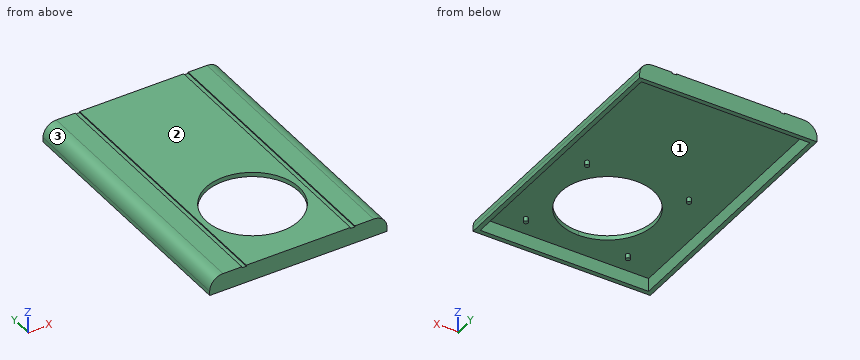
from build123d import *

# Parameters (mm, degrees)
F0_W      = 40
F0_H      = 60
F1_DEPTH  = 4
F2_W      = 1
F2_H      = 60
F3_DEPTH  = 0.25
F4_R      = 3
F6_DEPTH  = 25
F7_W      = 37.999998
F7_H      = 57.999999
F8_DEPTH  = 3
F10_DEPTH = 1


with BuildPart() as f1:
    # F0 (on Top) → F1 (new body)
    with BuildSketch(Plane.XY):
        with Locations((0, 3.187494)):
            Rectangle(F0_W, F0_H)
    extrude(amount=F1_DEPTH)

    # F2 (on face) → F3 (cut)
    with BuildSketch(Plane.XY.offset(4)):
        with Locations((-12.25, 3.187494)):
            Rectangle(F2_W, F2_H)
        with Locations((12.25, 3.187494)):
            Rectangle(F2_W, F2_H)
    extrude(amount=-F3_DEPTH, mode=Mode.SUBTRACT)

    # F4
    f4_edges = [f1.edges().sort_by_distance(p)[0] for p in [
        (-20, 3.187494, 4),
        (20, 3.187494, 4),
    ]]
    fillet(f4_edges, radius=F4_R)

    # F5 (on face) → F6 (cut)
    with BuildSketch(Plane.XY.offset(4)):
        with BuildLine():
            ThreePointArc((0, -20.812506), (7.424621, -17.737128), (10.5, -10.312506))
            ThreePointArc((10.5, -10.312506), (-7.424621, -2.887885), (0, -20.812506))
        make_face()
    extrude(amount=-F6_DEPTH, mode=Mode.SUBTRACT)

    # F7 (on face) → F8 (cut)
    with BuildSketch(Plane(origin=(0, 0, 0), x_dir=(1, 0, 0), z_dir=(0, 0, -1))):
        with Locations((0, -3.187493)):
            Rectangle(F7_W, F7_H)
    extrude(amount=-F8_DEPTH, mode=Mode.SUBTRACT)

    # F9 (on face) → F10 (join)
    with BuildSketch(Plane(origin=(0, 0, 3), x_dir=(1, 0, 0), z_dir=(0, 0, -1))):
        with BuildLine():
            Line((11.5, 21.312506), (11, 21.312506))
            ThreePointArc((11, 21.312506), (11.146447, 20.958953), (11.5, 20.812506))
            Line((11.5, 20.812506), (11.5, 21.312506))
        make_face()
        with BuildLine():
            ThreePointArc((12, 21.312506), (11.5, 21.812506), (11, 21.312506))
            Line((11, 21.312506), (11.5, 21.312506))
            Line((11.5, 21.312506), (11.5, 20.812506))
            ThreePointArc((11.5, 20.812506), (11.853553, 20.958953), (12, 21.312506))
        make_face()
        with BuildLine():
            Line((-11.5, 21.312506), (-11, 21.312506))
            ThreePointArc((-11, 21.312506), (-11.853553, 21.66606), (-11.5, 20.812506))
            Line((-11.5, 20.812506), (-11.5, 21.312506))
        make_face()
        with BuildLine():
            ThreePointArc((-11.5, 20.812506), (-11.146447, 20.958953), (-11, 21.312506))
            Line((-11, 21.312506), (-11.5, 21.312506))
            Line((-11.5, 21.312506), (-11.5, 20.812506))
        make_face()
        with BuildLine():
            Line((11.5, -0.687494), (11.5, -0.187494))
            ThreePointArc((11.5, -0.187494), (11.146447, -0.33394), (11, -0.687494))
            Line((11, -0.687494), (11.5, -0.687494))
        make_face()
        with BuildLine():
            ThreePointArc((12, -0.687494), (11.853553, -0.33394), (11.5, -0.187494))
            Line((11.5, -0.187494), (11.5, -0.687494))
            Line((11.5, -0.687494), (11, -0.687494))
            ThreePointArc((11, -0.687494), (11.5, -1.187494), (12, -0.687494))
        make_face()
        with BuildLine():
            ThreePointArc((-11, -0.687494), (-11.146447, -0.33394), (-11.5, -0.187494))
            Line((-11.5, -0.187494), (-11.5, -0.687494))
            Line((-11.5, -0.687494), (-11, -0.687494))
        make_face()
        with BuildLine():
            Line((-11.5, -0.687494), (-11.5, -0.187494))
            ThreePointArc((-11.5, -0.187494), (-11.853553, -1.041047), (-11, -0.687494))
            Line((-11, -0.687494), (-11.5, -0.687494))
        make_face()
    extrude(amount=F10_DEPTH)


solid = f1.part
Source: CAD feature listing. Evaluate the final solid. Frame: model axes, mm. Face numbers are marked on the shaded views. Round coordinates to 2 decimals unless told otherwise and drop trailing zeros. Loops run counter-clockwise (first coordinate to the right, second up) from the corner with the lowest first, then second, coordinate; pieces in that order, holes last. Notation, with made-up numbers: (78.5, 64.5) - (82.5, 64.5) arc R14 cw to (82.5, 78.5) - close; hole circle Ø3 at (48.25, -26). An arc over 180 degrees is marked (long way). Write item = value, one per line. Start each with the question number.
(1) Pull-direction query (X, two-part tool) for the marked faces 1, 2 and 3; classes: +X half, -X half, draft (parallel to the pull), parting line (faces both ways), or undercut.
(2) Pin query (flat end, axial travel): pin 1 (1.1 mm diameter, centred on x = 11.5, y = 0.5, fed in from -Z); pin 2 (0.8 mm diameter, centred on x = 12.5, y = 9.5, fed in from +Z). Return the tip coordinate at first contact, or that it passes through.
(3) Section query C-C, the plane x = -13.5. Output: boundary loops of the cut face in (y, z), plus the area to 3 significant figures.
(4) Ray query, line 1 along Y through (x, z) = (-11.5, 2.5); line 2 along Y through (x, z) = (-15.5, 1.5); line 3 along X through (y, z) = (17.5, 0.55). Return the intervals inside material, ascending. Write a range as from..to.
(5) Section query D-D, the plane y = -12.5. Output: boundary loops of the cut face in (x, z).
(6) Section query B-B, the plane x = 4.5. Output: boundary loops of the cut face in (y, z).
(7) Section query A-A, the plane y = -20. Output: boundary loops of the cut face in (x, z).
Conclusion:
q1.face_1 = undercut
q1.face_2 = draft
q1.face_3 = -X half
q2.pin_1 = 2
q2.pin_2 = 4
q3.outline = (-26.81, 0) - (-25.81, 0) - (-25.81, 3) - (32.19, 3) - (32.19, 0) - (33.19, 0) - (33.19, 4) - (-26.81, 4) - close
q3.area = 66.0 mm2
q4.line_1 = -26.81..-25.81, -21.81..-20.81, 0.19..1.19, 32.19..33.19
q4.line_2 = -26.81..-25.81, 32.19..33.19
q4.line_3 = -20..-19, 19..20
q5.outline = (-20, 0) - (-19, 0) - (-19, 3) - (-10.27, 3) - (-10.27, 4) - (-11.75, 4) - (-11.75, 3.75) - (-12.75, 3.75) - (-12.75, 4) - (-17, 4) arc R3 ccw to (-20, 1) - close; (10.27, 3) - (19, 3) - (19, 0) - (20, 0) - (20, 1) arc R3 ccw to (17, 4) - (12.75, 4) - (12.75, 3.75) - (11.75, 3.75) - (11.75, 4) - (10.27, 4) - close
q6.outline = (-26.81, 0) - (-25.81, 0) - (-25.81, 3) - (-19.8, 3) - (-19.8, 4) - (-26.81, 4) - close; (-0.83, 3) - (32.19, 3) - (32.19, 0) - (33.19, 0) - (33.19, 4) - (-0.83, 4) - close
q7.outline = (-20, 0) - (-19, 0) - (-19, 3) - (-4.05, 3) - (-4.05, 4) - (-11.75, 4) - (-11.75, 3.75) - (-12.75, 3.75) - (-12.75, 4) - (-17, 4) arc R3 ccw to (-20, 1) - close; (4.05, 3) - (19, 3) - (19, 0) - (20, 0) - (20, 1) arc R3 ccw to (17, 4) - (12.75, 4) - (12.75, 3.75) - (11.75, 3.75) - (11.75, 4) - (4.05, 4) - close
